The figure shows three views and two pictorial views of one solid part (mm, origin at its lowest corner). Answer the questions. A direction names the side the tool comes from. Give positions to 0.01 mm unless a question says otherwise; leave off trailing zeros. Loops run counter-clockwise (first coordinate to the right, second up) from the corner with the lowest first, then second, coordinate; pieces in that order, holes last. Notation, with made-up numbers: M -33.5,-16.5 L 20.5,-16.5 A8 cw 20.5,-4.5 Z; hole C -34.5,-27 d8. An arc over 180 degrees is marked long. Write item = value, one per line. Start each with the question number.
1. Section D-D on z = 8 is taken. Determine the outline of the cut face in (x, y).
2. Flat-ended cylindrical pins translate along their axes: pin 1 Ø4 at (x, z) = (14.5, 7.5) entering from +Y; pin 2 Ø5 at (x, y) = (11, 11) entering from -Z; pin 3 Ø1.6 at (x, z) = (26, 2.5) entering from -Y (1 decimal); pin 4 Ø4 at (y, z) = (6.5, 7) entering from +X. Find the tip coordinate at first contact, or state that the pin passes through.
3. The mould has two halves that part along Y. Classify the marked faces 1, 2, 3 and 4: released by +Y, released by -Y, zero draft, split by the parting line, or undercut.
4. Section B-B on x = 0.8 is taken. Determine the outline of the cut face in (y, z).
5. Section C-C on y = 4.25 is taken. Determine the outline of the cut face in (x, z).
6. For the marked faces 5, 6, 7, 8 and 9, determine the directions among +Z, -Z, +X, -X, +Y, -Y from which every point of the face is accessible in a straight line to the end or side of a thin tool.
7. Consider L1, parallel to Z at x = 17.5, y = 11.5; L2, parallel to Y at x = 1, z = 1; L3, parallel to Y at x = 8, z = 2.5 (1 decimal). Determine where each line is inside the solid, lowest interval first. Write a range as [from, to].
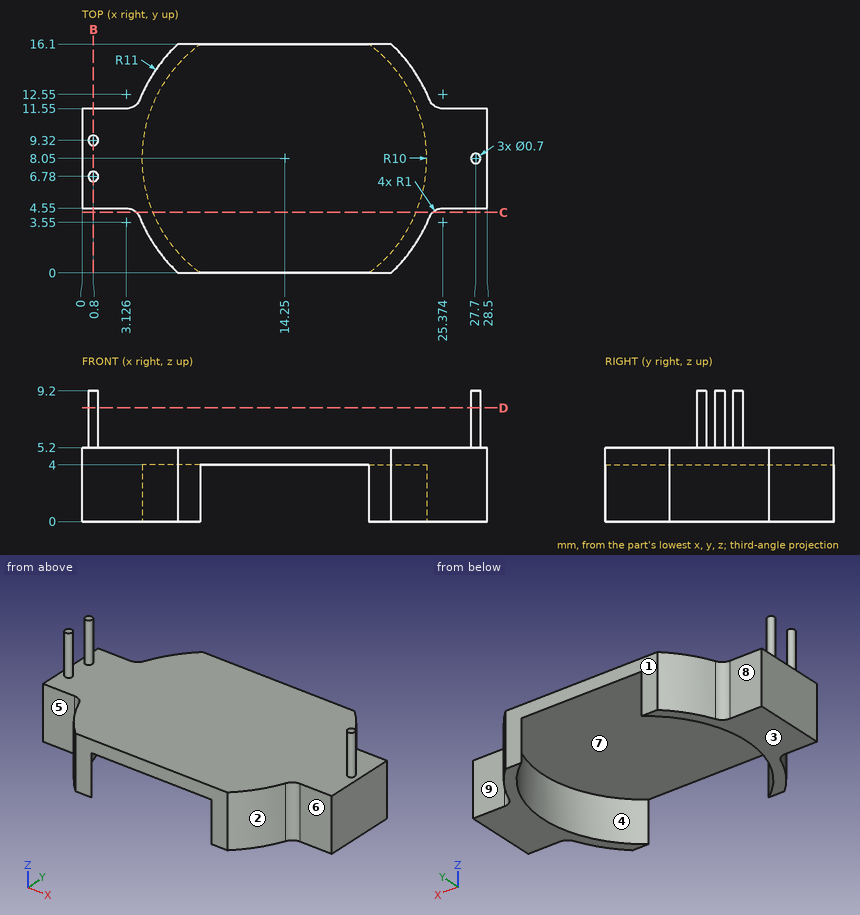
Verdict:
q1.outline = C 0.8,6.78 d0.7; C 0.8,9.32 d0.7; C 27.7,8.05 d0.7
q2.pin_1 = through
q2.pin_2 = 4
q2.pin_3 = 4.5
q2.pin_4 = 28.5
q3.face_1 = released by +Y
q3.face_2 = released by -Y
q3.face_3 = zero draft
q3.face_4 = undercut
q4.outline = M 4.55,0 L 11.55,0 L 11.55,5.2 L 9.67,5.2 L 9.67,9.2 L 8.97,9.2 L 8.97,5.2 L 7.13,5.2 L 7.13,9.2 L 6.43,9.2 L 6.43,5.2 L 4.55,5.2 Z
q5.outline = M 3.84,0 L 5,0 L 5,4 L 23.5,4 L 23.5,0 L 24.66,0 L 24.66,5.2 L 3.84,5.2 Z
q6.face_5 = +Z, -Z, -X, -Y
q6.face_6 = +Z, -Z, +X, -Y
q6.face_7 = -Z
q6.face_8 = +Z, -Z, -X, +Y
q6.face_9 = +Z, -Z, +X, +Y
q7.L1 = [4, 5.2]
q7.L2 = [4.55, 11.55]
q7.L3 = [0, 0.2], [15.9, 16.1]
